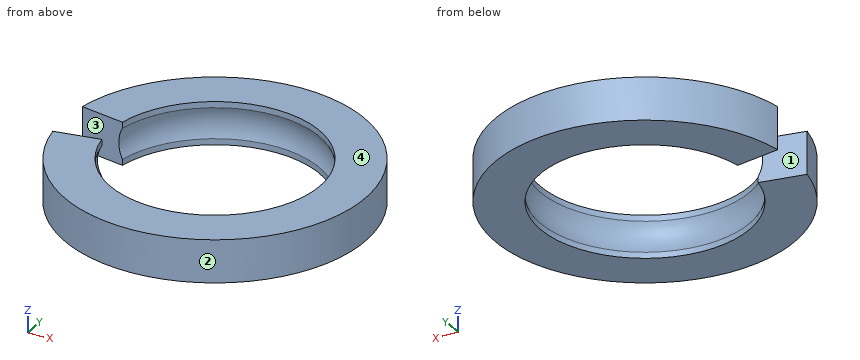
```python
from build123d import *

# Parameters (mm, degrees)
SKETCH1_R           = 22.5
SKETCH1_R_2         = 15.7
BOSS_EXTRUDE1_DEPTH = 6.4
CUT_EXTRUDE1_DEPTH  = 33.457048541


with BuildPart() as part:
    # Sketch1 → Boss-Extrude1 (new body)
    with BuildSketch(Plane.XY):
        Circle(SKETCH1_R)
        Circle(SKETCH1_R_2, mode=Mode.SUBTRACT)
    extrude(amount=BOSS_EXTRUDE1_DEPTH)

    # Sketch2 → Cut-Extrude1 (cut, through all)
    with BuildSketch(Plane.XY):
        Polygon((0, 0), (-29.645546143, 5.227309643), (-29.645546143, -5.227309643), align=None)
    extrude(amount=CUT_EXTRUDE1_DEPTH, mode=Mode.SUBTRACT)

    # Sketch5 → Cut-Revolve1 (revolve, cut)
    with BuildSketch(Plane(origin=(0, 0, 0), x_dir=(-0.984807753012197, 0.1736481776669938, 0), z_dir=(-0.1736481776669938, -0.984807753012197, 0))):
        with BuildLine():
            Line((15.7, -0.9), (15.7, -5.5))
            ThreePointArc((15.7, -5.5), (16.301238658, -3.2), (15.7, -0.9))
        make_face()
    revolve(axis=Axis((0, 0, -0.32), (0, 0, 1)), mode=Mode.SUBTRACT)


solid = part.part
```
Can you work these out from the model? Positions are in its coordinate system, mm. Face numbers are marked on the shaded views. Coordinates: 2 decimals unless noted, no trailing zeros. Loops run counter-clockwise (first coordinate to the right, second up) from the corner with the lowest first, then second, coordinate; pieces in that order, holes last.
Item 1: I'm going to push flat-ended pins straight in: pin 1 (3 mm diameter, centred on x = 9.5, z = 5, fed in from +Y); pin 2 (19 mm diameter, centred on x = 0, y = 0, fed in from -Z); pin 3 (1.5 mm diameter, centred on y = -5.5, z = 5, fed in from +X). Where does each tip first touch, or does it pass through?
Answers below:
pin 1: stops at y = 21.03
pin 2: passes through
pin 3: stops at x = 21.99
Item 2: Suppose I cut it at C-C (z = 3.75). Please give me the cut outline in (x, y), then the cut area to 3 significant figures.
Answers below:
outline: (-22.16, -3.91) arc R22.5 ccw (long way) to (-22.16, 3.91) - (-16.02, 2.83) arc R16.27 cw (long way) to (-16.02, -2.83) - close
area: 717 mm2
Item 3: Suppose I cut it at A-A (x = 0). Please give me the cut outline in (y, z).
Answers below:
outline: (-22.5, 0) - (-15.7, 0) - (-15.7, 0.9) arc R4.7 cw to (-15.7, 5.5) - (-15.7, 6.4) - (-22.5, 6.4) - close; (15.7, 0) - (22.5, 0) - (22.5, 6.4) - (15.7, 6.4) - (15.7, 5.5) arc R4.7 cw to (15.7, 0.9) - close
Item 4: Suppose I cut it at B-B (y = 0). Please give me the cut outline in (x, z).
Answers below:
outline: (15.7, 0) - (22.5, 0) - (22.5, 6.4) - (15.7, 6.4) - (15.7, 5.5) arc R4.7 cw to (15.7, 0.9) - close
Item 5: Please list where these lines run through material, in increasing order: L1, parallel to Y at x = 0, z = 0.45; L2, parallel to Y at x = -17, z = 6.25; L3, parallel to X at y = 9, z = 1.5.
Answers below:
L1: y = -22.5 to -15.7, 15.7 to 22.5
L2: y = -14.74 to -3, 3 to 14.74
L3: x = -20.62 to -13.21, 13.21 to 20.62
Item 6: If we mould it in two halves opening along Y, with no side actions, what happens to the marked faces 1, 2, 3 and 4? For each: released by +Y, released by -Y, zero draft, split by the parting line, or undercut.
Answers below:
face 1: undercut
face 2: split by the parting line
face 3: undercut
face 4: zero draft
